Geometry: final body of the model. Coordinates: model frame, mm. Give positions to 0.01 mm unless a question says otherwise; leave off trailing zeros. Write each loop counter-clockwise with the first axis right and the second up, starting at its lowest first coordinate (ties: lowest second). Pieces come first, ordered by that corner, then holes. Notation, with made-up numbers: M 17.5,-38 L 62.5,-38 A5 ccw 62.5,-30 Z; hole C 37.25,14.25 d1. An arc over 180 degrees is marked long. Use one line per item in the form item = value. Start each with the question number.
Item 1: Section query C-C on y = -2.25. Return loops of the section in (x, z), then the cut area to 3 significant figures.
Item 2: Pull-direction query (Y, two-part tool) for faces 1 (the cylindrical face through (-13.628, 0.049, 3.944)), 2 (the cylindrical face through (-6.797, -11.806, 3.944)), 3 (the cylindrical face through (0.672, -8.458, 3.944)); classes: released by +Y, released by -Y, zero draft, split by the parting line, or undercut.
Item 3: Section query B-B on x = 3. Return loops of the section in (y, z).
Item 4: Section query D-D on z = 2.5. Give the number of separate pieces and of enclosed holes in the cut face, then the cut area to 3 significant figures.
Item 5: Material intervals for line 1 along Y through (x, z) = (0, 4); line 2 along Y through (x, z) = (-0.75, 7.25); line 3 along X through (y, z) = (1.25, 6.5), sorted ascending. Write a range as from..to.
Item 6: Contact query for flat-ended pins moving along their axis: P1, Ø2, axis at x = 5.5, y = -3, coming from the -Z side; P2, Ø4, axis at x = -6.5, z = 1.5, coming from the -Y side; P3, Ø2, axis at y = 9, z = 6, coming from the +X side. Output: stop coordinate, or through.
Item 7: Section query A-A on x = 0. Return loops of the section in (y, z).
from build123d import *

# Parameters (mm, degrees)
SKETCH1_R           = 4.7625
SKETCH1_R_2         = 1.25
BOSS_EXTRUDE1_DEPTH = 8


with BuildPart() as part:
    # Sketch1 → Boss-Extrude1 (new body)
    with BuildSketch(Plane.XY):
        with BuildLine():
            Line((-13.253372163, -1.044486042), (-7.531237528, -10.955513958))
            ThreePointArc((-7.531237528, -10.955513958), (-6.784217233, -11.816359568), (-5.770008435, -12.336431676))
            Line((-5.770008435, -12.336431676), (-0.836847118, -13.76941319))
            ThreePointArc((-0.836847118, -13.76941319), (0, -13.888495471), (0.836847118, -13.76941319))
            Line((0.836847118, -13.76941319), (5.770008435, -12.336431676))
            ThreePointArc((5.770008435, -12.336431676), (6.784217233, -11.816359568), (7.531237528, -10.955513958))
            Line((7.531237528, -10.955513958), (13.253372163, -1.044486042))
            ThreePointArc((13.253372163, -1.044486042), (13.625376182, 0.032875315), (13.568667441, 1.171241953))
            Line((13.568667441, 1.171241953), (12.343085176, 6.159975731))
            ThreePointArc((12.343085176, 6.159975731), (12.027789898, 6.944247736), (11.506238058, 7.609437458))
            Line((11.506238058, 7.609437458), (7.798659006, 11.165189723))
            ThreePointArc((7.798659006, 11.165189723), (6.841158949, 11.783484253), (5.722134635, 12))
            Line((5.722134635, 12), (-5.722134635, 12))
            ThreePointArc((-5.722134635, 12), (-6.841158949, 11.783484253), (-7.798659006, 11.165189723))
            Line((-7.798659006, 11.165189723), (-11.506238058, 7.609437458))
            ThreePointArc((-11.506238058, 7.609437458), (-12.027789898, 6.944247736), (-12.343085176, 6.159975731))
            Line((-12.343085176, 6.159975731), (-13.568667441, 1.171241953))
            ThreePointArc((-13.568667441, 1.171241953), (-13.625376182, 0.032875315), (-13.253372163, -1.044486042))
        make_face()
        Circle(SKETCH1_R, mode=Mode.SUBTRACT)
        with Locations((-8.238066653, 4.75625)):
            Circle(SKETCH1_R_2, mode=Mode.SUBTRACT)
        with Locations((8.238066653, 4.75625)):
            Circle(SKETCH1_R_2, mode=Mode.SUBTRACT)
        with Locations((0, -9.5125)):
            Circle(SKETCH1_R_2, mode=Mode.SUBTRACT)
    extrude(amount=BOSS_EXTRUDE1_DEPTH)


solid = part.part
Answer sheet:
q1.outline = M -12.56,0 L -4.2,0 L -4.2,8 L -12.56,8 Z; M 4.2,0 L 12.56,0 L 12.56,8 L 4.2,8 Z
q1.area = 134 mm2
q2.face_1 = split by the parting line
q2.face_2 = released by -Y
q2.face_3 = undercut
q3.outline = M -13.14,0 L -3.7,0 L -3.7,8 L -13.14,8 Z; M 3.7,0 L 12,0 L 12,8 L 3.7,8 Z
q4.separate_pieces = 1
q4.enclosed_holes = 4
q4.area = 453 mm2
q5.line_1 = -13.89..-10.76, -8.26..-4.76, 4.76..12
q5.line_2 = -13.79..-10.51, -8.51..-4.7, 4.7..12
q5.line_3 = -13.55..-4.6, 4.6..13.55
q6.P1 = 0
q6.P2 = -12.71
q6.P3 = 11.1
q7.outline = M -13.89,0 L -10.76,0 L -10.76,8 L -13.89,8 Z; M -8.26,0 L -4.76,0 L -4.76,8 L -8.26,8 Z; M 4.76,0 L 12,0 L 12,8 L 4.76,8 Z
